from build123d import *

# Parameters (mm, degrees)
BOSS_EXTRU_1_START = 1.5
BOSS_EXTRU_1_DEPTH = 4
CHANFREIN1_SIZE    = 1
CHANFREIN1_SIZE2   = 2
ESQUISSE3_W        = 0.4
ESQUISSE3_H        = 2
BOSS_EXTRU_2_DEPTH = 5


with BuildPart() as part:
    # Esquisse1 → Révolution1 (revolve)
    with BuildSketch(Plane.XY, mode=Mode.PRIVATE) as r_volution1_sk:
        with BuildLine():
            Line((4.4, 4.340153416), (4.4, 2))
            Line((4.4, 2), (7, 2))
            Line((7, 2), (7, 0))
            Line((7, 0), (6.35, 0))
            Line((6.35, 0), (6.35, -7))
            Line((6.35, -7), (5.5, -7))
            Line((5.5, -7), (5.5, -9))
            Line((5.5, -9), (4.25, -9))
            Line((4.25, -9), (4.25, -15.1))
            Line((4.25, -15.1), (0, -15.1))
            Line((0, -15.1), (0, 5))
            ThreePointArc((0, 5), (2.224600948, 4.834121161), (4.4, 4.340153416))
        make_face()
    revolve(r_volution1_sk.sketch.rotate(Axis((0, 15.574511932, 0), (0, -1, 0)), 90), axis=Axis((0, 15.574511932, 0), (0, -1, 0)))

    # Esquisse2 → Boss.-Extru.1 (add)
    with BuildSketch(Plane.XZ.offset(BOSS_EXTRU_1_START)):
        Polygon((4.618802154, -8), (9.237604307, 0), (4.618802154, 8), (-4.618802154, 8), (-9.237604307, 0), (-4.618802154, -8), align=None)
    extrude(amount=BOSS_EXTRU_1_DEPTH)

    # Chanfrein1
    chanfrein1_edges = [part.edges().sort_by_distance(p)[0] for p in [
        (0, 2, -7),
    ]]
    chanfrein1_side = [part.faces().sort_by_distance(p)[0] for p in [
        (0, 1, -7),
    ]]
    chamfer(chanfrein1_edges, length=CHANFREIN1_SIZE, length2=CHANFREIN1_SIZE2, reference=chanfrein1_side[0])

    # Esquisse3 → Boss.-Extru.2 (add)
    with BuildSketch(Plane.XZ.offset(15.1)):
        with Locations((-2, 0)):
            Rectangle(ESQUISSE3_W, ESQUISSE3_H)
    boss_extru_2 = extrude(amount=BOSS_EXTRU_2_DEPTH)

    # Symétrie1: Boss.-Extru.2 across plane
    add(boss_extru_2.mirror(Plane(origin=(0, 0, 0), x_dir=(0, 0, 1), z_dir=(1, 0, 0))))


solid = part.part
Here's how the part is built. I have some questions about the finished solid (model axes, mm). A direction names the side the tool comes from. Give positions to 0.01 mm unless a question says otherwise; leave off trailing zeros. Order: outer loops, then holes, each group sorted by start corner. A loop starts at its lowest first (then second) coordinate and runs counter-clockwise, first axis right, second up. Notation, with made-up numbers: M 4,14 L 55,14 A20 ccw 55,30 Z; hole C 3,19.5 d8. An arc over 180 degrees is marked long. Answer as a JSON object with one key per item and string values. Group by question number.
1) I'm going to push flat-ended pins straight in: pin 1 Ø1 at (y, z) = (-5, 3) entering from +X; pin 2 Ø1.5 at (x, z) = (7, 3.5) entering from +Y; pin 3 Ø6 at (x, z) = (-0.5, -3) entering from +Y; pin 4 Ø2 at (y, z) = (-17.5, -0.5) entering from +X. Where does each tip first touch, or does it pass through?
2) We'd pull the mould along X, two halves only. Please class faces 1 (the flat face through (3, -5.5, -6)), 2 (the flat face through (6.896, -3.472, -4.056)), 3 (the flat face through (1.8, -18, 0)): pulls with the +X half, pulls with the -X half, needs draft (parallel to the pull), parting line crosses it, or undercut.
3) Suppose I cut it at D-D, the plane y = 3.25. Write out the boundary of the cut face in (x, z).
4) On a 3-axis mill with a long thin cutter (end or side, diameter ignored), from which of +Z, -Z, +X, -X, +Y, -Y can I reach the whole of each face in a straight line? I mean faces 4 (the flat face through (-2.2, -18, 0)), 5 (the cylindrical face through (-4.363, 3.154, -0.573)), 6 (the cylindrical face through (3.86, -0.76, -5.04)), 7 (the cylindrical face through (5.37, -8.01, -1.19)). Say none if no direction works.
5) Suppose I cut it at C-C, the plane y = -5. Write out the boundary of the cut face in (x, z).
6) Suppose I cut it at A-A, the plane y = -18. Write out the boundary of the cut face in (x, z), plus the area to 3 significant figures.
7) Please list where these lines run through material, in increasing order: L1, parallel to X at y = -16, z = -0.5; L2, parallel to Y at x = -4, z = -7; L3, parallel to X at y = -15, z = 0. Write a range as [from, to].
Results found:
{
 "1": {"pin 1": "x = 7.79", "pin 2": "y = -1.5", "pin 3": "y = 5", "pin 4": "x = 2.2"},
 "2": {"face 1": "needs draft", "face 2": "pulls with the +X half", "face 3": "undercut"},
 "3": {"outline": "C 0,0 d8.8"},
 "4": {"face 4": "+Z, -Z, -X, -Y", "face 5": "+Y", "face 6": "none", "face 7": "-Y"},
 "5": {"outline": "M -9.24,0 L -4.62,-8 L 4.62,-8 L 9.24,0 L 4.62,8 L -4.62,8 Z"},
 "6": {"outline": "M -2.2,-1 L -1.8,-1 L -1.8,1 L -2.2,1 Z; M 1.8,-1 L 2.2,-1 L 2.2,1 L 1.8,1 Z", "area": "1.60 mm²"},
 "7": {"L1": "[-2.2, -1.8], [1.8, 2.2]", "L2": "[-5.5, -1.5]", "L3": "[-4.25, 4.25]"}
}
